Autodesk Fusion 360 part; units mm, degrees
sketch "Sketch1" plane through (0, 0, 0) normal (0, 1, 0) x (1, 0, 0)
  line L0 (-30, 0) -> (30, 0)
  line L1 (30, 0) -> (30, -4)
  line L2 (30, -4) -> (-30, -4)
  line L3 (-30, -4) -> (-30, 0)
  line L4 (-18, -4) -> (-11.2, -4)
  line L5 (-11.2, -4) -> (-11.2, -24)
  line L6 (-11.2, -24) -> (-18, -24)
  line L7 (-18, -24) -> (-18, -4)
  circle A0 centre (-14.1, -20) radius 1
  line L8 (0, -20) -> (0, -2.5)
  line L9 (11.2, -24) -> (18, -24)
  line L10 (11.2, -4) -> (11.2, -24)
  line L11 (18, -24) -> (18, -4)
  circle A1 centre (14.1, -20) radius 1
  dimension "d1" = 4
  dimension "d2" = 60
  dimension "d3" = 6.8
  dimension "d4" = 30
  dimension "d5" = 18
  dimension "d6" = 20
  dimension "d7" = 2
  dimension "d8" = 2.9
  dimension "d9" = 4
  dimension "d10" = 4
extrude "Extrude1" add sketch "Sketch1" along normal blind 12 contours L0 L1 L2 L3 L4
extrude "Extrude2" add sketch "Sketch1" along normal blind 9 and the other way blind -3 contours L2 L4 L5 L6 L7 | L2 L9 L10 L11
chamfer "Chamfer1" distance 5 angle 45 2 edges at (-11.2, 6, 4) (11.2, 6, 4)
sketch "Sketch2" plane through (0, 0, 0) normal (0, 0, 1) x (1, 0, 0)
  circle A0 centre (-24, 6) radius 2
  line L0 (0, 2.5) -> (0, 20)
  circle A1 centre (24, 6) radius 2
  dimension "d18" = 4
  dimension "d19" = 24
  dimension "d20" = 6
extrude "Extrude3" cut sketch "Sketch2" along normal blind 10
fillet "Fillet1" radius 6 4 edges at (-30, 0, 2) (30, 0, 2) (30, 12, 2) (-30, 12, 2)
equation "d4 = d2 / 2"
equation "d10 = d1"
Geometry: final body of the model. Coordinates: model frame, mm. A direction names the side the tool comes from. Coordinates: 2 decimals unless noted, no trailing zeros. Order: outer loops, then holes, each group sorted by start corner. A loop starts at its lowest first (then second) coordinate and runs counter-clockwise, first axis right, second up. Notation, with made-up numbers: M -17,-9 L 23,-9 A32 cw 23,23 Z; hole C 62,61.25 d4. An arc over 180 degrees is marked long. One line per question, with ' | ' between items. Start each with the question number.
Item 1: Cut plane B-B, the plane x = 14.1. Return the cut outline in (y, z), then the cut area to 3 significant figures.
Item 2: Draft query along Z for faces 1 (the cylindrical face through (28.196, 1.711, 2.028)), 2 (the cylindrical face through (14.56, 5.96, 19.11)), 3 (the flat face through (15, 6, 24)). Return one class per face: released by +Z, released by -Z, zero draft, split by the parting line, or undercut.
Item 3: Ray query, probe 1 along X at (y, z) = (6, 1.3); probe 2 along X at (y, z) = (4.95, 20); probe 3 along Z at (x, y) = (14.1, 7.3). Return the intervals inside material, ascending. Write a range as [from, to].
Item 4: Set-up query: faces 4 (the flat face through (8.7, 6, 6.5)), 5 (the flat face through (-15, 3, 14)), 6 (the flat face through (0, 6, 4)). Return all of +Z, -Z, +X, -X, +Y, -Y with unobstructed straight access to the full face (end or side cutting, diameter ignored); none if empty.
Item 5: Cut plane A-A, the plane z = 7.25. Return the cut outline in (x, y), then the cut area to 3 significant figures.
Item 6: Pin query (flat end, axial travel): pin 1 Ø6.5 at (x, y) = (-24, 6) entering from +Z; pin 2 Ø6.5 at (y, z) = (4.5, 10.5) entering from +X; pin 3 Ø5 at (x, z) = (-17.5, 11) entering from +Y. Return the tip coordinate at first contact, or that it passes through.
Item 7: Cut plane C-C, the plane z = 9.75. Return the cut outline in (x, y), then the cut area to 3 significant figures.
Item 8: Cut plane D-D, the plane x = -9. Return the cut outline in (y, z).
A:
1) outline: M 0,0 L 12,0 L 12,4 L 9,4 L 9,19 L 3,19 L 3,4 L 0,4 Z; M 3,21 L 9,21 L 9,24 L 3,24 Z | area: 156 mm2
2) face 1: zero draft | face 2: undercut | face 3: released by +Z
3) probe 1: x = [-30, -26], [-22, 22], [26, 30] | probe 2: x = [-18, -15.1], [-13.1, -11.2], [11.2, 13.1], [15.1, 18] | probe 3: z = [0, 19], [21, 24]
4) face 4: +Z, +Y, -Y | face 5: +Z, +X, -X, -Y | face 6: +Z
5) outline: M -18,3 L -9.45,3 L -9.45,9 L -18,9 Z; M 9.45,3 L 18,3 L 18,9 L 9.45,9 Z | area: 103 mm2
6) pin 1: stops at z = 4 | pin 2: stops at x = 18 | pin 3: stops at y = 9
7) outline: M -18,3 L -11.2,3 L -11.2,9 L -18,9 Z; M 11.2,3 L 18,3 L 18,9 L 11.2,9 Z | area: 81.6 mm2
8) outline: M 0,0 L 12,0 L 12,4 L 9,4 L 9,6.8 L 3,6.8 L 3,4 L 0,4 Z
